Study the drawing (mm; zero at the part's minimum x, y, z) and answer. A direction names the side the tool comes from. Coordinates: 2 decimals unless noted, no trailing zeros. Loops run counter-clockwise (first coordinate to the right, second up) from the corner with the lowest first, then second, coordinate; pieces in that order, holes last. Notation, with made-up numbers: (23, 25.25) - (55, 25.25) arc R21 cw to (55, 33.25) - close; hole circle Ø7 at (-31.75, 1.5). An arc over 180 degrees is marked (long way). Use one line per item in the form item = value.
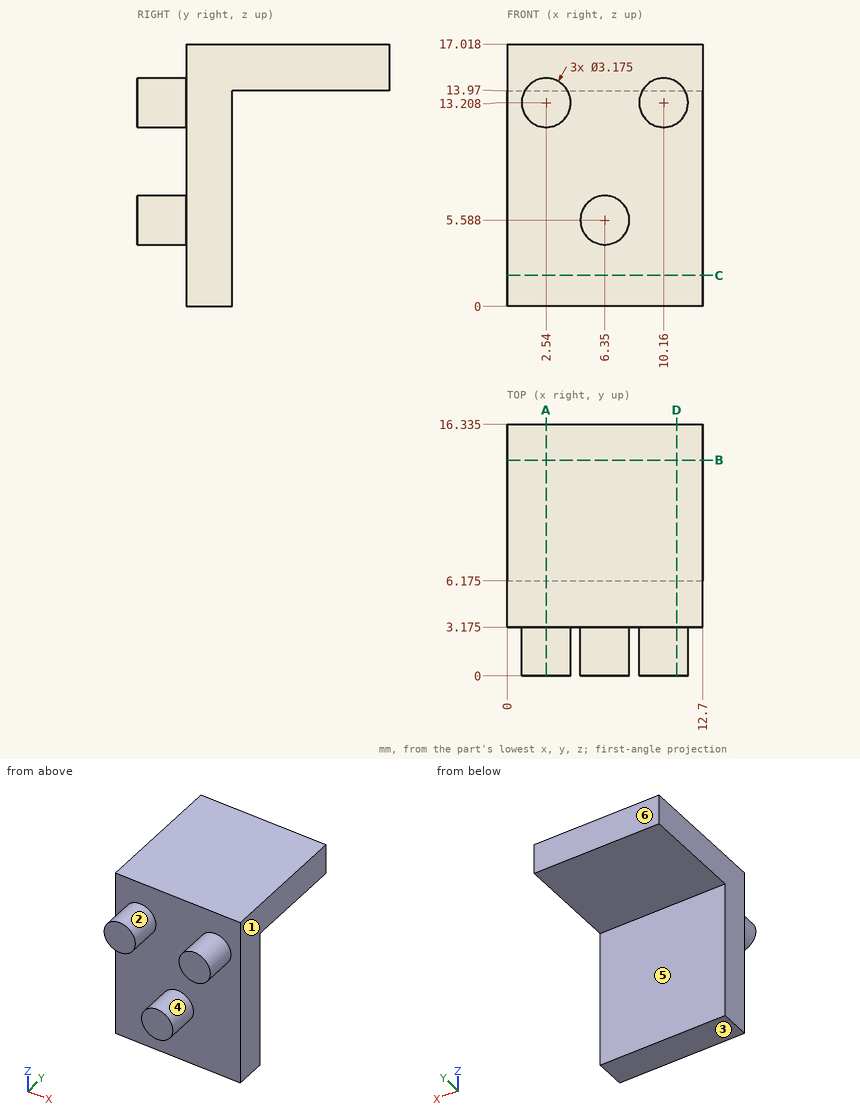
Item 1: Which of the six approach directions +Z, -Z, +X, -X, +Y, -Y give full straight-line access (tool end or side, diameter ignored) to the marked faces 4, 5 and 6?
Results below:
face_4 = -Y
face_5 = -Z, +X, -X, +Y
face_6 = +Z, -Z, +X, -X, +Y
Item 2: The part is cut by section A-A on x = 2.54. Give the vertices of the cut face in (y, z) (1 decimal).
Results below:
outline = (0, 11.6) - (3.2, 11.6) - (3.2, 0) - (6.2, 0) - (6.2, 14) - (16.3, 14) - (16.3, 17) - (3.2, 17) - (3.2, 14.8) - (0, 14.8) - close
Item 3: Each of these flat-tipped pins is pushed along its axis until it touches: P1, Ø1, axis at x = 3.5, z = 7, coming from the -Y side (3 decimals); P2, Ø3, axis at x = 9.5, y = 10.5, coming from the -Z side. Where does it stop, or does it pass through?
Results below:
P1 = 3.175
P2 = 13.97
Item 4: The part is cut by section D-D on x = 11. Give the vertices of the cut face in (y, z) (3 decimals), plus the area to 3 significant figures.
Results below:
outline = (0, 11.861) - (3.175, 11.861) - (3.175, 0) - (6.175, 0) - (6.175, 13.97) - (16.335, 13.97) - (16.335, 17.018) - (3.175, 17.018) - (3.175, 14.555) - (0, 14.555) - close
area = 90.6 mm²
Item 5: The part is cut by section B-B on y = 14. Give the vertices of the cut face in (x, z), plus the area to 3 significant figures.
Results below:
outline = (0, 13.97) - (12.7, 13.97) - (12.7, 17.02) - (0, 17.02) - close
area = 38.7 mm²
Item 6: For a pull along X with two mould halves and no side action, classify the marked faces 1, 2 and 3 as +X half, -X half, draft (parallel to the pull), parting line (faces both ways), or undercut.
Results below:
face_1 = +X half
face_2 = undercut
face_3 = draft
Item 7: The part is cut by section C-C on z = 2. Give the vertices of the cut face in (x, y) (3 decimals), plus the area to 3 significant figures.
Results below:
outline = (0, 3.175) - (12.7, 3.175) - (12.7, 6.175) - (0, 6.175) - close
area = 38.1 mm²
Item 8: Find the intervals of material crossed by L1, parallel to Y at x = 11.25, z = 5 (3 decimals); L2, parallel to Z at x = 7.25, y = 11.75; L3, parallel to Y at x = 5.5, z = 14 (3 decimals), in increasing order.
Results below:
L1 = 3.175 to 6.175
L2 = 13.97 to 17.02
L3 = 3.175 to 16.335
